Could you check a few things on this model? Use its own coordinates, in mm. Give positions to 0.01 mm unless a question says otherwise; leave off trailing zeros. Write each loop counter-clockwise with the first axis right and the second up, starting at its lowest first coordinate (ties: lowest second). Pieces come first, ordered by that corner, then holes. Notation, with made-up numbers: (-19, -39.5) - (40, -39.5) arc R15 cw to (40, -26.5) - close; hole circle Ø1 at (48.25, 13). An arc over 180 degrees is marked (long way). Use one line per item in the form item = value.
```python
from build123d import *

# Parameters (mm, degrees)
SKETCH1_W           = 163.57
SKETCH1_H           = 20
SKETCH1_R           = 1
BOSS_EXTRUDE1_DEPTH = 5
SKETCH2_R           = 1.6
CUT_EXTRUDE1_DEPTH  = 2
SKETCH3_R           = 1.5
CUT_EXTRUDE2_DEPTH  = 10


with BuildPart() as part:
    # Sketch1 → Boss-Extrude1 (new body)
    with BuildSketch(Plane(origin=(0, 0, 0), x_dir=(1, 0, 0), z_dir=(0, 1, 0))):
        Rectangle(SKETCH1_W, SKETCH1_H)
        with Locations((-79.825, 6)):
            Circle(SKETCH1_R, mode=Mode.SUBTRACT)
        with Locations((-79.825, -6)):
            Circle(SKETCH1_R, mode=Mode.SUBTRACT)
        with Locations((79.825, 6)):
            Circle(SKETCH1_R, mode=Mode.SUBTRACT)
        with Locations((79.825, -6)):
            Circle(SKETCH1_R, mode=Mode.SUBTRACT)
    extrude(amount=BOSS_EXTRUDE1_DEPTH)

    # Sketch2 → Cut-Extrude1 (cut)
    with BuildSketch(Plane(origin=(0, 5, 0), x_dir=(1, 0, 0), z_dir=(0, 1, 0))):
        with Locations((-79.825, 6)):
            Circle(SKETCH2_R)
        with Locations((-79.825, -6)):
            Circle(SKETCH2_R)
        with Locations((79.825, 6)):
            Circle(SKETCH2_R)
        with Locations((79.825, -6)):
            Circle(SKETCH2_R)
    extrude(amount=-CUT_EXTRUDE1_DEPTH, mode=Mode.SUBTRACT)

    # Sketch3 → Cut-Extrude2 (cut)
    with BuildSketch(Plane(origin=(0, 5, 0), x_dir=(1, 0, 0), z_dir=(0, 1, 0))):
        with Locations((-25, 0)):
            Circle(SKETCH3_R)
        with Locations((25, 0)):
            Circle(SKETCH3_R)
    extrude(amount=-CUT_EXTRUDE2_DEPTH, mode=Mode.SUBTRACT)


solid = part.part
```
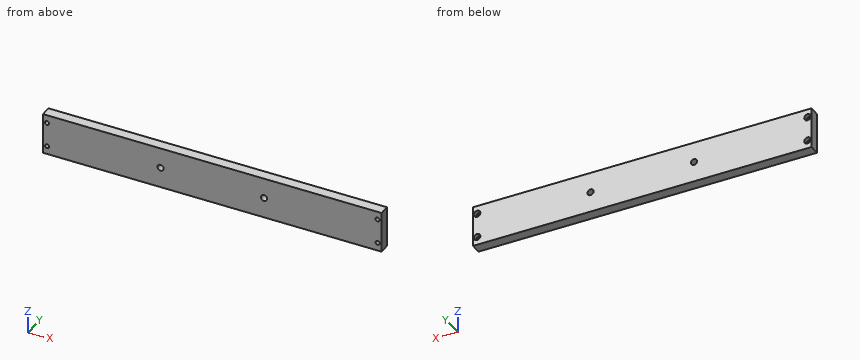
1. Imagine slicing it at A-A, the plane z = 0. List the corners of the cut face in (x, y) for me (3 decimals).
Response values:
outline = (-81.785, 0) - (-26.5, 0) - (-26.5, 5) - (-81.785, 5) - close; (-23.5, 0) - (23.5, 0) - (23.5, 5) - (-23.5, 5) - close; (26.5, 0) - (81.785, 0) - (81.785, 5) - (26.5, 5) - close
2. If I drill on line 1 (X direction, y = 2.05, z = 6) (3 decimals); line 2 (X direction, y = 3.2, z = 0) (3 decimals); line 3 (Z direction, x = 25, y = 3.45), over which ranges is the centre line in solid material (lowest first)? Write a range as from..to.
Response values:
line_1 = -81.785..-80.825, -78.825..78.825, 80.825..81.785
line_2 = -81.785..-26.5, -23.5..23.5, 26.5..81.785
line_3 = -10..-1.5, 1.5..10
3. Imagine slicing it at B-B, the plane x = 25. List the corners of the cut face in (y, z) for me.
Response values:
outline = (0, -10) - (5, -10) - (5, -1.5) - (0, -1.5) - close; (0, 1.5) - (5, 1.5) - (5, 10) - (0, 10) - close
4. For pin 1 (2.5 mm diameter, centred on x = 79.825, z = -6, fed in from +Y), with a flat end and sliding along its axis, tell me the tip position at first contact or that it passes through.
Response values:
pin_1 = 3
